Here's how the part is built. I have some questions about the finished solid (model axes, mm). Round coordinates to 2 decimals unless told otherwise and drop trailing zeros. Write each loop counter-clockwise with the first axis right and the second up, starting at its lowest first coordinate (ties: lowest second). Pieces come first, ordered by that corner, then holes. Notation, with made-up numbers: (-14.5, 57.5) -> (-9.5, 57.5) arc R27 cw to (-9.5, 83.5) -> close; hole circle Ø6 at (84, 53.25). An arc over 180 degrees is marked (long way). Answer in a Markdown table with one row per item. Add a question column.
Autodesk Inventor part; units mm, degrees
ref_plane "Work Plane1" through (-32.8309, 24, 0) normal (0, 1, 0) x (-1, 0, 0)
ref_plane "YZ Plane" through (0, 0, 0) normal (1, 0, 0) x (0, 1, 0)
ref_plane "XZ Plane" through (0, 0, 0) normal (0, 1, 0) x (-1, 0, 0)
sketch "Sketch1" plane through (0, 0, 0) normal (0, 0, 1) x (1, 0, 0)
  arc A0 (-38.8309, 24) -> (-26.8309, 24) centre (-32.8309, 24) ccw
  arc A1 (-37.8309, 24) -> (-27.8309, 24) centre (-32.8309, 24) ccw
  line L0 (-38.8309, 24) -> (-26.8309, 24)
  point P0 (0, 0)
  dimension "d0" = 1
  dimension "d1" = 5
ref_plane "Work Plane1" through (-32.8309, 24, 0) normal (0, 1, 0) x (-1, 0, 0)
sketch "Sketch2" plane through (-32.8309, 24, 0) normal (0, 1, 0) x (-1, 0, 0)
  point P0 (-32.8309, 0)
extrude "Extrusion1" add sketch "Sketch1" along normal blind 1 contours L0 A1 A0
sketch "Sketch3" plane through (-27.8309, 24, 0) normal (0, 1, 0) x (1, 0, 0)
  line L0 (1, 0) -> (0, 0)
  line L1 (0, 0) -> (0, -1)
  line L2 (1, -1) -> (0, -1)
  line L3 (1, 0) -> (1, -1)
  line L4 (0.1, -0.1) -> (0.9, -0.1)
  line L5 (0.9, -0.1) -> (0.9, -0.9)
  line L6 (0.9, -0.9) -> (0.1, -0.9)
  line L7 (0.1, -0.9) -> (0.1, -0.1)
  point P0 (27.8309, 0)
  dimension "d4" = 0.8
extrude "Extrusion2" add sketch "Sketch3" along normal blind 1 contours L4 L5 L6 L7
properties part number "McCrea_kabel_walle"
Item 1: If we section it at B-B on y = 21.75: Please give me the cut outline in (x, z).
Item 2: I need wall thicknesses on line 1 along X through (y, z) = (22.5, 0.2); line 2 along X through (y, z) = (23.75, 0.6); line 3 along X through (y, z) = (24.5, 0.45). Which ranges of each line are inside material? Lowest first, please. Write a range as from..to.
Item 3: If we section it at C-C on y = 23.5: Please give me the cut outline in (x, z).
Item 4: If we section it at D-D on x = -28: Please give me the cut outline in (y, z).
Item 5: For P1, Ø0.6, axis at x = -27, y = 24.5, coming from the -Z side; P2, Ø0.6, axis at x = -27, y = 24.5, coming from the +Z side; P3, Ø0.5, axis at x = -38.5, z = 0.5, coming from the +Y side, each with a flat end and sliding along its axis, tell me the tip position at first contact or that it passes through.
Item 6: If we section it at A-A on z = 0.75: Please give me the cut outline in (x, y).
Item 7: If we mould it in two halves opening along X, with no side actions, what happens to faces 1 (the cylindrical face through (-32.7, 18, 0.5)), 2 (the flat face through (-38.3, 24, 0.5)), 3 (the cylindrical face through (-32.7, 19, 0.5))? For each: pulls with the +X half, pulls with the -X half, needs draft (parallel to the pull), parting line crosses it, or undercut.
Results list:
| question | item | result |
|---|---|---|
| 1 | outline | (-38.39, 0) -> (-37.3, 0) -> (-37.3, 1) -> (-38.39, 1) -> close; (-28.37, 0) -> (-27.27, 0) -> (-27.27, 1) -> (-28.37, 1) -> close |
| 2 | line 1 | -38.64..-37.6, -28.06..-27.02 |
| 2 | line 2 | -38.83..-37.82, -27.84..-26.84 |
| 2 | line 3 | -27.73..-26.93 |
| 3 | outline | (-38.81, 0) -> (-37.81, 0) -> (-37.81, 1) -> (-38.81, 1) -> close; (-27.86, 0) -> (-26.85, 0) -> (-26.85, 1) -> (-27.86, 1) -> close |
| 4 | outline | (20.44, 0) -> (22.71, 0) -> (22.71, 1) -> (20.44, 1) -> close |
| 5 | P1 | z = 0.1 |
| 5 | P2 | z = 0.9 |
| 5 | P3 | y = 24 |
| 6 | outline | (-38.83, 24) arc R6 ccw to (-26.83, 24) -> (-26.93, 24) -> (-26.93, 25) -> (-27.73, 25) -> (-27.73, 24) -> (-27.83, 24) arc R5 cw to (-37.83, 24) -> close |
| 7 | face 1 | parting line crosses it |
| 7 | face 2 | needs draft |
| 7 | face 3 | undercut |
